The listing builds one solid part. Answer for the finished solid, in the listing's coordinates (mm). A direction names the side the tool comes from. Coordinates: 2 decimals unless noted, no trailing zeros. Loops run counter-clockwise (first coordinate to the right, second up) from the corner with the lowest first, then second, coordinate; pieces in that order, holes last. Notation, with made-up numbers: (40, 18) - (89, 18) arc R17 ccw to (89, 23) - close; hole circle Ø9 at (-35, 49.5). An arc over 180 degrees is marked (long way). Put each result on its own line as item: value.
```python
from build123d import *

# Parameters (mm, degrees)
SKETCH_1_R      = 50
EXTRUDE_1_DEPTH = 60
EXTRUDE_START   = 22
SKETCH_2_R      = 3
EXTRUDE_2_DEPTH = 10
EXTRUDE_START_2 = -18
SKETCH_3_W      = 62
SKETCH_3_H      = 35
EXTRUDE_3_DEPTH = 10
FILLET_1_R      = 5
SKETCH_4_R      = 5
EXTRUDE_4_DEPTH = 6


with BuildPart() as part:
    # 草图1 → 凸台-拉伸1 (new body)
    with BuildSketch(Plane(origin=(0, 0, 0), x_dir=(1, 0, 0), z_dir=(0, 1, 0))):
        with Locations(Location((0, 0, 0), (0, 0, 90))):
            Circle(SKETCH_1_R)
    extrude(amount=EXTRUDE_1_DEPTH)

    # 草图2 → 凸台-拉伸2 (add)
    with BuildSketch(Plane.XY.offset(EXTRUDE_START)):
        with BuildLine():
            Line((38, 60), (38, 95))
            Line((38, 95), (-24, 95))
            Line((-24, 95), (-24, 96))
            ThreePointArc((-24, 96), (-32, 104), (-40, 96))
            Line((-40, 96), (-40, 90))
            Line((-40, 90), (-22.679491924, 60))
            Line((-22.679491924, 60), (38, 60))
        make_face()
        with Locations((-32, 96)):
            Circle(SKETCH_2_R, mode=Mode.SUBTRACT)
    extrude(amount=EXTRUDE_2_DEPTH)

    # 草图3 → 凸台-拉伸3 (add)
    with BuildSketch(Plane.XY.offset(EXTRUDE_START_2)):
        with Locations((7, 77.5)):
            Rectangle(SKETCH_3_W, SKETCH_3_H)
    extrude(amount=-EXTRUDE_3_DEPTH)

    # 圆角1
    fillet_1_edges = [part.edges().sort_by_distance(p)[0] for p in [
        (38, 95, 27),
        (38, 95, -23),
        (-24, 95, -23),
    ]]
    fillet(fillet_1_edges, radius=FILLET_1_R)

    # 草图4 → 凸台-拉伸4 (add, symmetric)
    with BuildSketch(Plane.XY):
        with BuildLine():
            Line((12.880830473, 87.733418669), (5, 60))
            Line((5, 60), (40, 60))
            Line((40, 60), (32.119169527, 87.733418669))
            ThreePointArc((32.119169527, 87.733418669), (22.5, 95), (12.880830473, 87.733418669))
        make_face()
        with Locations((22.5, 85)):
            Circle(SKETCH_4_R, mode=Mode.SUBTRACT)
    extrude(amount=EXTRUDE_4_DEPTH, both=True)


solid = part.part
```
1) The part is cut by section A-A (z = 0). Give the vertices of the cut face in (x, y), and give its area (3 significant figures).
Found:
outline: (-50, 0) - (50, 0) - (50, 60) - (40, 60) - (32.12, 87.73) arc R10 ccw to (12.88, 87.73) - (5, 60) - (-50, 60) - close; hole circle Ø10 at (22.5, 85)
area: 6,780 mm^2
2) The part is cut by section D-D (x = 22.5). Give the vertices of the cut face in (y, z).
Found:
outline: (0, -44.65) - (60, -44.65) - (60, -28) - (95, -28) - (95, -18) - (60, -18) - (60, -6) - (80, -6) - (80, 6) - (60, 6) - (60, 22) - (95, 22) - (95, 32) - (60, 32) - (60, 44.65) - (0, 44.65) - close; (90, -6) - (95, -6) - (95, 6) - (90, 6) - close
3) Each of these flat-tipped pins is pushed along its axis until it touches: pin 1 (8 mm diameter, centred on x = 22.5, y = 85, fed in from -Z); pin 2 (0.5 mm diameter, centred on y = 95.5, z = 25, fed in from +X); pin 3 (8 mm diameter, centred on y = 79, z = -22.5, fed in from -X). Where does it stop, or does it pass through?
Found:
pin 1: stops at z = -28
pin 2: stops at x = -24
pin 3: stops at x = -24
4) The part is cut by section C-C (x = 0). Give the vertices of the cut face in (y, z), and give its area (3 significant figures).
Found:
outline: (0, -50) - (60, -50) - (60, -28) - (95, -28) - (95, -18) - (60, -18) - (60, 22) - (95, 22) - (95, 32) - (60, 32) - (60, 50) - (0, 50) - close
area: 6,700 mm^2
5) For a pull along Z with two mould halves and no side action, classify faces 1 (the face through (-1, 0, 1)), 2 (the face through (-2, 77, 22)), 3 (the face through (22, 74, 6)), 4 (the face through (-15.02, 29.58, -47.69)) as pulls with the +Z half, pulls with the -Z half, needs draft (parallel to the pull), parting line crosses it, or undercut.
Found:
face 1: needs draft
face 2: undercut
face 3: undercut
face 4: parting line crosses it
6) Straight lines are drawn through the part: L1, parallel to Z at x = 34, y = 81; L2, parallel to Z at x = 0.5, y = 65; L3, parallel to Y at x = -32, z = 25.25. For each, find the intervals that lie inside material, in ascending order. Write a range as [from, to].
Found:
L1: z = [-28, -18], [-6, 6], [22, 32]
L2: z = [-28, -18], [22, 32]
L3: y = [0, 60], [76.14, 93], [99, 104]
7) The part is cut by section B-B (y = 77.5). Give the vertices of the cut face in (x, z).
Found:
outline: (-32.78, 22) - (38, 22) - (38, 32) - (-32.78, 32) - close; (-24, -28) - (38, -28) - (38, -18) - (-24, -18) - close; (9.97, -6) - (35.03, -6) - (35.03, 6) - (9.97, 6) - close
8) For faces 5 (the face through (5, 95, 27)), 6 (the face through (-24, 75, -23)), 7 (the face through (8.996, 74.061, 0.084)), 8 (the face through (36.115, 73.673, 0.084)), determine the directions among +Z, -Z, +X, -X, +Y, -Y from which every point of the face is accessible in a straight line to the end or side of a thin tool.
Found:
face 5: +Z, -Z, +X, +Y
face 6: -Z, -X, +Y
face 7: -X, +Y
face 8: +X, +Y
